Check sheet for the drawn part. Datum: minimum x, y, z corner. Units: mm. A direction names the side the tool comes from. Give positions to 0.01 mm unless a question says otherwise; leave off trailing zeros. Loops run counter-clockwise (first coordinate to the right, second up) from the corner with the lowest first, then second, coordinate; pieces in that order, holes last.
1. Cross-section at B-B, the plane y = 2.5. Record the cut outline in (x, z).
2. Cross-section at D-D, the plane x = 8. Record the cut outline in (y, z).
3. Cross-section at A-A, the plane z = 3.25. Record the cut outline in (x, y).
4. Go/stop test with flat-tipped pins: pin 1 Ø2 at (y, z) = (7.5, 32) entering from +X; pin 2 Ø4 at (x, y) = (7, 7) entering from -Z; pin 3 Ø8 at (x, z) = (7.5, 9.5) entering from -Y. Record where each tip stops, or that it passes through.
5. Release check for a two-part mould opening along Z. For the marked faces 1, 2 and 3 record: +Z half, -Z half, draft (parallel to the pull), parting line (faces both ways), or undercut.
6. Cross-section at C-C, the plane x = 13. Record the cut outline in (y, z).
7. Material ranges on L1, parallel to Z at x = 7, y = 1.75; L2, parallel to Z at x = 3, y = 10.5; L3, parallel to Y at x = 2, z = 11.5, recorded low to high.
8. Tool access check on the marked faces 4 and 5. Record the directions out of +Z, -Z, +X, -X, +Y, -Y that give a thin tool (end or side, any length) a straight path to the whole face; none if there is none.
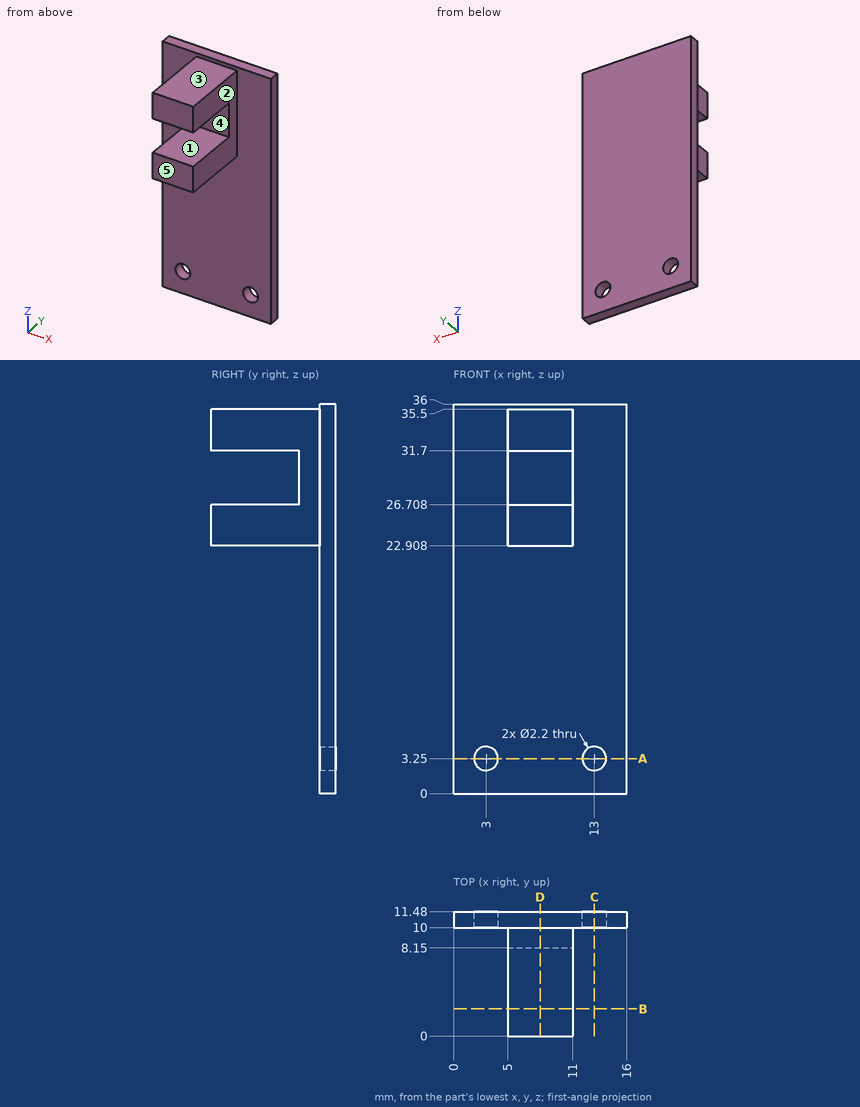
Result:
1. outline: (5, 22.91) - (11, 22.91) - (11, 26.71) - (5, 26.71) - close; (5, 31.7) - (11, 31.7) - (11, 35.5) - (5, 35.5) - close
2. outline: (0, 22.91) - (10, 22.91) - (10, 0) - (11.48, 0) - (11.48, 36) - (10, 36) - (10, 35.5) - (0, 35.5) - (0, 31.7) - (8.15, 31.7) - (8.15, 26.71) - (0, 26.71) - close
3. outline: (0, 10) - (1.9, 10) - (1.9, 11.48) - (0, 11.48) - close; (4.1, 10) - (11.9, 10) - (11.9, 11.48) - (4.1, 11.48) - close; (14.1, 10) - (16, 10) - (16, 11.48) - (14.1, 11.48) - close
4. pin 1: stops at x = 11
4. pin 2: stops at z = 22.91
4. pin 3: stops at y = 10
5. face 1: undercut
5. face 2: draft
5. face 3: +Z half
6. outline: (10, 0) - (11.48, 0) - (11.48, 2.15) - (10, 2.15) - close; (10, 4.35) - (11.48, 4.35) - (11.48, 36) - (10, 36) - close
7. L1: z = 22.91 to 26.71, 31.7 to 35.5
7. L2: z = 0 to 2.15, 4.35 to 36
7. L3: y = 10 to 11.48
8. face 4: +X, -X, -Y
8. face 5: +Z, -Z, +X, -X, -Y
